Could you check a few things on this model? Use its own coordinates, in mm. A direction names the side the tool comes from. Coordinates: 2 decimals unless noted, no trailing zeros. Order: outer loops, then holes, each group sorted by start corner. A loop starts at its lowest first (then second) coordinate and runs counter-clockwise, first axis right, second up. Notation, with made-up numbers: M -26.75,-34 L -17.75,-34 A25 ccw -17.75,-19 Z; hole C 22.5,1.25 d10. An arc over 180 degrees is marked long. Put each result on its own line as item: value. Start each with the question number.
Autodesk Inventor part; units mm, degrees
ref_plane "YZ Plane" through (0, 0, 0) normal (1, 0, 0) x (0, 1, 0)
sketch "Sketch2" plane through (0, 0, 0) normal (1, 0, 0) x (0, 1, 0)
  line L0 (0, 19) -> (0, 29)
  line L1 (0, 29) -> (1.5, 29)
  line L2 (1.5, 29) -> (1.5, 20.5)
  line L3 (0, 19) -> (13.5, 19)
  line L4 (14, 18.5) -> (14, 0)
  line L5 (1.5, 20.5) -> (13.5, 20.5)
  line L6 (15.5, 18.5) -> (15.5, 0)
  line L7 (-3.1828, 0) -> (19.0971, 0)
  line L8 (0, -40.6) -> (0, 40.6)
  line L9 (0, -19) -> (0, -29)
  line L10 (0, -29) -> (1.5, -29)
  line L11 (1.5, -29) -> (1.5, -20.5)
  line L12 (0, -19) -> (14, -19)
  line L13 (14, -19) -> (14, 0)
  line L14 (1.5, -20.5) -> (13.5, -20.5)
  line L15 (15.5, -18.5) -> (15.5, 0)
  arc A0 (15.5, 18.5) -> (13.5, 20.5) centre (13.5, 18.5) ccw
  arc A1 (13.5, -20.5) -> (15.5, -18.5) centre (13.5, -18.5) ccw
  arc A2 (14, 18.5) -> (13.5, 19) centre (13.5, 18.5) ccw
  point P0 (0, 0)
  point P1 (14, 19)
  point P2 (15.5, 20.5)
  point P3 (15.5, -20.5)
  point P4 (0, 26.5)
  point P5 (2.5, -19)
  point P6 (0, 19)
  dimension "d0" = 10
  dimension "d1" = 1.5
  dimension "d2" = 8.5
  dimension "d4" = 14
  dimension "d5" = 19
  dimension "d6" = 1.5
  dimension "d7" = 2
  dimension "d22" = 0.5
extrude "Extrusion1" add sketch "Sketch2" along normal mid plane 44 contours L0 L1 L2 L5 A0 L6 L7 L4 A2 L3 | L7 L15 A1 L14 L11 L10 L8 L12 L13
sketch "Sketch3" plane through (-22, 0, 19) normal (0, -1, 0) x (1, 0, 0)
  line L0 (0, 10) -> (44, 10)
  line L1 (22, -59.6) -> (22, 21.6)
  point P0 (22, -19)
  point P1 (22, 5)
  point P2 (39, 5)
  point P3 (5, 5)
  dimension "d10" = 5
  dimension "d12" = 17
  dimension "d14" = 5
  dimension "d23" = 17
  dimension "d24" = 5
hole "Hole1" at (0, 0, 24) at (17, 0, 24) at (-17, 0, 24) direction (0, 1, 0) diameter 4.2 end through all
mirror "Mirror1" about plane through (0, 0, 0) normal (0, 0, 1) of "Hole1"
properties part number "connector-houseing-top-cover"
Item 1: If we section it at C-C on z = 24: Write out the boundary of the cut face in (x, y).
Item 2: If we section it at B-B on x = -17: Write out the boundary of the cut face in (y, z).
Item 3: For faces 4 (the flat face through (0, 1.5, -27)), 5 (the flat face through (0, 14, 0)), 6 (the cylindrical face through (0.631, 0.76, -21.997)), 7 (the flat face through (0, 7, 20.5)), which set-ups out of +Z, -Z, +X, -X, +Y, -Y let a thin tool reach every point of the face, with its end or its side?
Item 4: If we mould it in two halves opening along X, with no side actions, what happens to faces 1 (the cylindrical face through (-18.77, 0.76, 22.87)), 2 (the flat face through (-22, 15, 0)), 3 (the flat face through (0, 15.5, 0))? For each: released by +X, released by -X, zero draft, split by the parting line, or undercut.
Item 5: I need wall thicknesses on probe 1 along Z at (x, y) = (0, 0.4); probe 2 along X at (y, z) = (0.9, 24); probe 3 along Z at (x, y) = (3, 5.75). Which ranges of each line are inside material? Lowest first, please.
Item 6: For pin 1 Ø1.5 at (x, y) = (15.5, 9.5) entering from +Z; pin 2 Ø4 at (x, z) = (-2.5, 23.5) entering from +Y; pin 3 Ø3.5 at (x, z) = (-17, -24) entering from +Y; pin 4 Ø3 at (x, y) = (-0.5, 6) entering from -Z, each with a flat end and sliding along its axis, tell me the tip position at first contact or that it passes through.
Item 7: If we section it at A-A on y = 9: Write out the boundary of the cut face in (x, z).
Item 8: If we section it at D-D on x = -3: Write out the boundary of the cut face in (y, z), then the cut area to 3 significant figures.
Geometry check:
1. outline: M -22,0 L -19.1,0 L -19.1,1.5 L -22,1.5 Z; M -14.9,0 L -2.1,0 L -2.1,1.5 L -14.9,1.5 Z; M 2.1,0 L 14.9,0 L 14.9,1.5 L 2.1,1.5 Z; M 19.1,0 L 22,0 L 22,1.5 L 19.1,1.5 Z
2. outline: M 0,-29 L 1.5,-29 L 1.5,-26.1 L 0,-26.1 Z; M 0,-21.9 L 1.5,-21.9 L 1.5,-20.5 L 13.5,-20.5 A2 ccw 15.5,-18.5 L 15.5,18.5 A2 ccw 13.5,20.5 L 1.5,20.5 L 1.5,21.9 L 0,21.9 L 0,19 L 13.5,19 A0.5 cw 14,18.5 L 14,-19 L 0,-19 Z; M 0,26.1 L 1.5,26.1 L 1.5,29 L 0,29 Z
3. face 4: -Z, +X, -X, +Y
3. face 5: +X, -X, -Y
3. face 6: +Y, -Y
3. face 7: +Z, +X, -X, +Y
4. face 1: undercut
4. face 2: released by -X
4. face 3: zero draft
5. probe 1: z = -29 to -26.1, -21.9 to -19, 19 to 21.9, 26.1 to 29
5. probe 2: x = -22 to -19.1, -14.9 to -2.1, 2.1 to 14.9, 19.1 to 22
5. probe 3: z = -20.5 to -19, 19 to 20.5
6. pin 1: stops at z = 20.5
6. pin 2: stops at y = 1.5
6. pin 3: passes through
6. pin 4: stops at z = -20.5
7. outline: M -22,-20.5 L 22,-20.5 L 22,-19 L -22,-19 Z; M -22,19 L 22,19 L 22,20.5 L -22,20.5 Z
8. outline: M 0,-29 L 1.5,-29 L 1.5,-20.5 L 13.5,-20.5 A2 ccw 15.5,-18.5 L 15.5,18.5 A2 ccw 13.5,20.5 L 1.5,20.5 L 1.5,29 L 0,29 L 0,19 L 13.5,19 A0.5 cw 14,18.5 L 14,-19 L 0,-19 Z
8. area: 127 mm²
